Read the model definition and answer for the solid it produces. Units are mm, in the model's axes. Face numbers are marked on the shaded views. Round coordinates to 2 decimals unless told otherwise and drop trailing zeros. Order: outer loops, then holes, each group sorted by start corner. A loop starts at its lowest first (then second) coordinate and runs counter-clockwise, first axis right, second up. Notation, with made-up numbers: (37.25, 23) - (81.25, 23) arc R29 cw to (81.25, 45) - close; hole circle Ø8 at (65.5, 46). An arc over 180 degrees is marked (long way). Put each result on its own line as item: value. Start each with the question number.
Q1. Find the intervals of material crossed by line 1 along Z through (x, y) = (0, 202.5); line 2 along Y through (x, z) = (-99, 129.5), in increasing order. Write a range as from..to.
Q2. For a pull along X with two mould halves and no side action, classify the marked faces 1, 2 and 3 as pulls with the +X half, pulls with the -X half, needs draft (parallel to the pull), parting line crosses it, or undercut.
Q3. Section C-C on z = 12.5 is taken. Give the vertices of the cut face in (x, y).
Q4. Section A-A on x = -23 is taken. Give the vertices of the cut face in (y, z), then the cut area to 3 significant figures.
Q5. Section D-D on z = 123 is taken. Give the vertices of the cut face in (x, y).
Q6. Section B-B on y = 101 is taken. Give the vertices of the cut face in (x, z), then the cut area to 3 significant figures.
Q7. Each of these flat-tipped pins is pushed along its axis until it touches: pin 1 Ø10 at (y, z) = (45.5, 38.5) entering from +X; pin 2 Ø2 at (x, z) = (72, 40) entering from +Y; pin 3 Ø4 at (y, z) = (200.5, -30.5) entering from +X. Where does it stop, or does it pass through?
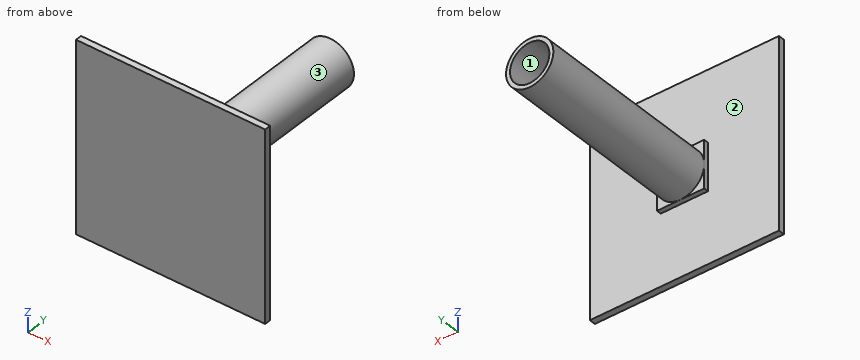
from build123d import *

# Parameters (mm, degrees)
SKETCH1_R           = 38.1
SKETCH1_R_2         = 31.75
BOSS_EXTRUDE1_DEPTH = 304.8
SKETCH2_W           = 76.2
SKETCH2_H           = 76.2
BOSS_EXTRUDE2_DEPTH = 7.62
SKETCH4_W           = 304.8
SKETCH4_H           = 304.8
BOSS_EXTRUDE4_DEPTH = 10.16


with BuildPart() as part:
    # Sketch1 → Boss-Extrude1 (new body)
    with BuildSketch(Plane(origin=(0, 0, 0), x_dir=(1, 0, 0), z_dir=(0, 1, 0))):
        Circle(SKETCH1_R)
        Circle(SKETCH1_R_2, mode=Mode.SUBTRACT)
    extrude(amount=BOSS_EXTRUDE1_DEPTH)

    # Sketch2 → Boss-Extrude2 (add)
    with BuildSketch(Plane(origin=(0, 0, 0), x_dir=(1, 0, 0), z_dir=(0, 1, 0))):
        Rectangle(SKETCH2_W, SKETCH2_H)
    extrude(amount=-BOSS_EXTRUDE2_DEPTH)

    # Sketch4 → Boss-Extrude4 (add)
    with BuildSketch(Plane(origin=(0, -7.62, 0), x_dir=(1, 0, 0), z_dir=(0, 1, 0))):
        Rectangle(SKETCH4_W, SKETCH4_H)
    extrude(amount=-BOSS_EXTRUDE4_DEPTH)


solid = part.part
Findings:
1. line 1: -38.1..-31.75, 31.75..38.1
1. line 2: -17.78..-7.62
2. face 1: undercut
2. face 2: needs draft
2. face 3: parting line crosses it
3. outline: (-152.4, -17.78) - (152.4, -17.78) - (152.4, -7.62) - (38.1, -7.62) - (38.1, 0) - (35.99, 0) - (35.99, 304.8) - (29.19, 304.8) - (29.19, 0) - (-29.19, 0) - (-29.19, 304.8) - (-35.99, 304.8) - (-35.99, 0) - (-38.1, 0) - (-38.1, -7.62) - (-152.4, -7.62) - close
4. outline: (-17.78, -152.4) - (-7.62, -152.4) - (-7.62, -38.1) - (0, -38.1) - (0, -30.37) - (304.8, -30.37) - (304.8, -21.89) - (0, -21.89) - (0, 21.89) - (304.8, 21.89) - (304.8, 30.37) - (0, 30.37) - (0, 38.1) - (-7.62, 38.1) - (-7.62, 152.4) - (-17.78, 152.4) - close
4. area: 8,850 mm2
5. outline: (-152.4, -17.78) - (152.4, -17.78) - (152.4, -7.62) - (-152.4, -7.62) - close
6. outline: circle Ø76.2 at (0, 0); hole circle Ø63.5 at (0, 0)
6. area: 1,390 mm2
7. pin 1: x = 18.15
7. pin 2: y = -7.62
7. pin 3: x = 25.29
